Verification items for the finished model (mm, model axes). Face numbers are marked on the shaded views. Round coordinates to 2 decimals unless told otherwise and drop trailing zeros. Order: outer loops, then holes, each group sorted by start corner. A loop starts at its lowest first (then second) coordinate and runs counter-clockwise, first axis right, second up. Notation, with made-up numbers: (28, 88.25) -> (62, 88.25) arc R21 ccw to (62, 92.25) -> close; hole circle Ø5 at (-26, -15). An arc over 180 degrees is marked (long way). Put each result on its own line as item: value.
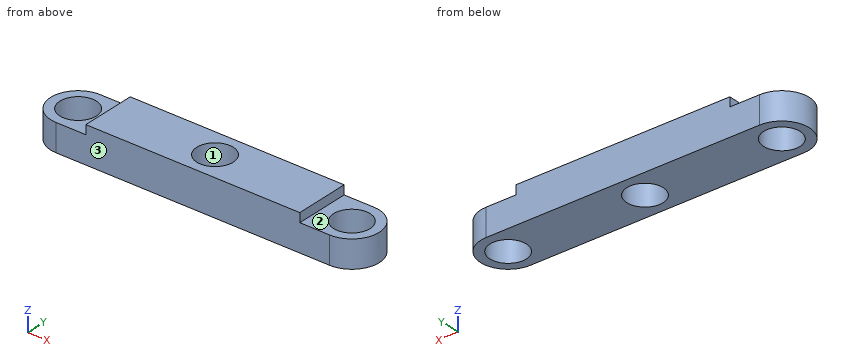
```python
from build123d import *

# Parameters (mm, degrees)
SKETCH_1_R          = 10
EXTRUDE_1_DEPTH     = 10
SKETCH_2_W          = 35.259791695
SKETCH_2_H          = 30
CUT_EXTRUDE_1_DEPTH = 5


with BuildPart() as part:
    # Эскиз1 → Бобышка-Вытянуть1 (new, symmetric)
    with BuildSketch(Plane.XY):
        with BuildLine():
            Line((-75, 15), (75, 15))
            ThreePointArc((75, 15), (90, 0), (75, -15))
            Line((75, -15), (-75, -15))
            ThreePointArc((-75, -15), (-90, 0), (-75, 15))
        make_face()
        with Locations((-75, 0)):
            Circle(SKETCH_1_R, mode=Mode.SUBTRACT)
        Circle(SKETCH_1_R, mode=Mode.SUBTRACT)
        with Locations((75, 0)):
            Circle(SKETCH_1_R, mode=Mode.SUBTRACT)
    extrude(amount=EXTRUDE_1_DEPTH, both=True)

    # Эскиз2 → Вырез-Вытянуть1 (cut)
    with BuildSketch(Plane.XY.offset(10)):
        with Locations((-76.250006928, 0)):
            Rectangle(SKETCH_2_W, SKETCH_2_H)
        with Locations((76.250006928, 0)):
            Rectangle(SKETCH_2_W, SKETCH_2_H)
    extrude(amount=-CUT_EXTRUDE_1_DEPTH, mode=Mode.SUBTRACT)


solid = part.part
```
Item 1: Material ranges on line 1 along Y through (x, z) = (-0.5, 7.75); line 2 along X through (y, z) = (6, 3); line 3 along X through (y, z) = (4, -3.5), recorded low to high.
Geometry check:
line 1: -15 to -9.99, 9.99 to 15
line 2: -88.75 to -83, -67 to -8, 8 to 67, 83 to 88.75
line 3: -89.46 to -84.17, -65.83 to -9.17, 9.17 to 65.83, 84.17 to 89.46
Item 2: Sectioned sample at C-C, the plane z = -5.5. Record the boundary of the cut face in (x, y).
Geometry check:
outline: (-75, -15) -> (75, -15) arc R15 ccw to (75, 15) -> (-75, 15) arc R15 ccw to start; hole circle Ø20 at (-75, 0); hole circle Ø20 at (0, 0); hole circle Ø20 at (75, 0)
Item 3: Sectioned sample at D-D, the plane z = 6.75. Record the boundary of the cut face in (x, y), then the cut area to 3 significant figures.
Geometry check:
outline: (-58.62, -15) -> (58.62, -15) -> (58.62, 15) -> (-58.62, 15) -> close; hole circle Ø20 at (0, 0)
area: 3,200 mm2
Item 4: Sectioned sample at B-B, the plane x = 0. Record the boundary of the cut face in (y, z).
Geometry check:
outline: (-15, -10) -> (-10, -10) -> (-10, 10) -> (-15, 10) -> close; (10, -10) -> (15, -10) -> (15, 10) -> (10, 10) -> close
Item 5: Depth check by flat-ended pin: pin 1 Ø3 at (y, z) = (5, 5) entering from -X; pin 2 Ø4 at (y, z) = (4, -2.5) entering from -X; pin 3 Ø4 at (y, z) = (-7, 7.5) entering from -X. Enter the tip coordinate at first touch or a pass-through.
Geometry check:
pin 1: x = -89.59
pin 2: x = -89.87
pin 3: x = -58.62
Item 6: Release check for a two-part mould opening along Y. For the marked faces 1, 2 and 3 record: pulls with the +Y half, pulls with the -Y half, needs draft (parallel to the pull), parting line crosses it, or undercut.
Geometry check:
face 1: undercut
face 2: needs draft
face 3: pulls with the -Y half
Item 7: Sectioned sample at A-A, the plane y = 0. Record the boundary of the cut face in (x, z).
Geometry check:
outline: (-90, -10) -> (-85, -10) -> (-85, 5) -> (-90, 5) -> close; (-65, -10) -> (-10, -10) -> (-10, 10) -> (-58.62, 10) -> (-58.62, 5) -> (-65, 5) -> close; (10, -10) -> (65, -10) -> (65, 5) -> (58.62, 5) -> (58.62, 10) -> (10, 10) -> close; (85, -10) -> (90, -10) -> (90, 5) -> (85, 5) -> close
